Geometry check sheet. Reference: drawing and pictorial views, mm from the part's lowest x, y, z. Coordinates: 2 decimals unless noted, no trailing zeros. Loops run counter-clockwise (first coordinate to the right, second up) from the corner with the lowest first, then second, coordinate; pieces in that order, holes last. Notation, with made-up numbers: (79.5, 24) -> (99.5, 24) arc R16 ccw to (99.5, 40) -> close; hole circle Ø9 at (71, 35.5). An arc over 180 degrees is marked (long way). Answer as a JSON object with one key per item and string values. Group by question number.
Q1. Gauge pin test, flat ends, axial feed: pin 1 Ø2.5 at (x, y) = (45, 9) entering from +Z; pin 2 Ø3 at (x, y) = (45, 21) entering from +Z. Record the tip position at first contact, or that the pin passes through.
Q2. Cross-section at C-C on y = 3. Record the boundary of the cut face in (x, z), and give its area (3 significant figures).
Q3. Cross-section at A-A on y = 21. Record the boundary of the cut face in (x, z), and give its area (3 significant figures).
Q4. Scan lines: L1, parallel to Y at x = 45, z = 0.35; L2, parallel to X at y = 21, z = 0.5; L3, parallel to Y at x = 25, z = 0.5. Record each from-to range of solid material in increasing order.
Q5. Cross-section at B-B on z = 0.35. Record the boundary of the cut face in (x, y).
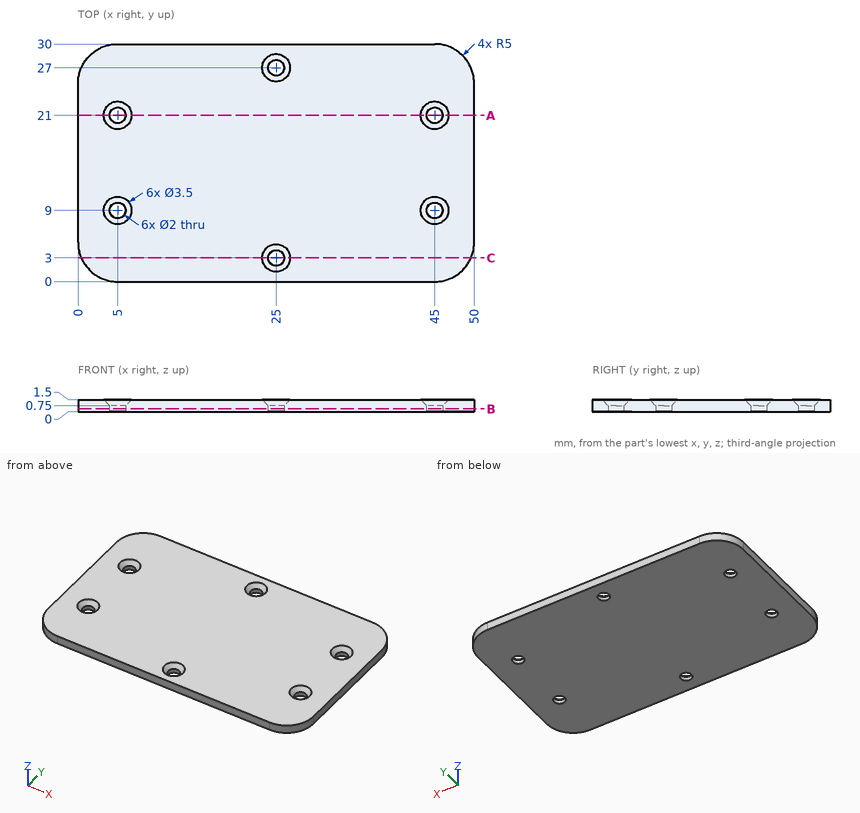
Computed values:
{
 "1": {"pin 1": "stops at z = 1", "pin 2": "stops at z = 1.25"},
 "2": {"outline": "(0.42, 0) -> (24, 0) -> (24, 0.75) -> (23.25, 1.5) -> (0.42, 1.5) -> close; (26, 0) -> (49.58, 0) -> (49.58, 1.5) -> (26.75, 1.5) -> (26, 0.75) -> close", "area": "70.2 mm²"},
 "3": {"outline": "(0, 0) -> (4, 0) -> (4, 0.75) -> (3.25, 1.5) -> (0, 1.5) -> close; (6, 0) -> (44, 0) -> (44, 0.75) -> (43.25, 1.5) -> (6.75, 1.5) -> (6, 0.75) -> close; (46, 0) -> (50, 0) -> (50, 1.5) -> (46.75, 1.5) -> (46, 0.75) -> close", "area": "67.9 mm²"},
 "4": {"L1": "y = 0 to 8, 10 to 20, 22 to 30", "L2": "x = 0 to 4, 6 to 44, 46 to 50", "L3": "y = 0 to 2, 4 to 26, 28 to 30"},
 "5": {"outline": "(0, 5) arc R5 ccw to (5, 0) -> (45, 0) arc R5 ccw to (50, 5) -> (50, 25) arc R5 ccw to (45, 30) -> (5, 30) arc R5 ccw to (0, 25) -> close; hole circle Ø2 at (5, 9); hole circle Ø2 at (5, 21); hole circle Ø2 at (25, 3); hole circle Ø2 at (25, 27); hole circle Ø2 at (45, 9); hole circle Ø2 at (45, 21)"}
}
